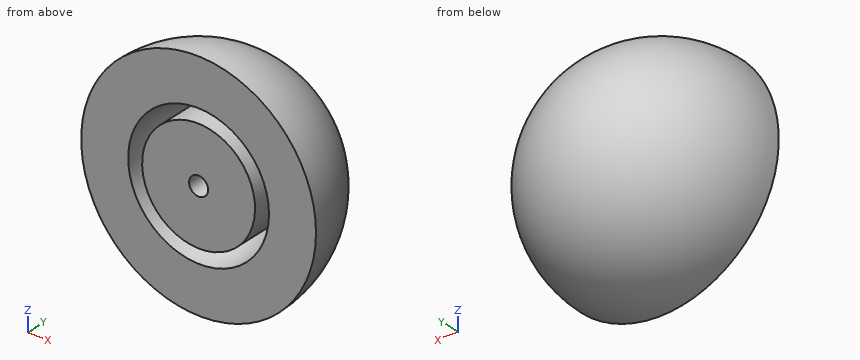
Autodesk Inventor part; units mm, degrees
ref_plane "YZ Plane" through (0, 0, 0) normal (1, 0, 0) x (0, 1, 0)
ref_plane "XZ Plane" through (0, 0, 0) normal (0, 1, 0) x (-1, 0, 0)
ref_plane "XY Plane" through (0, 0, 0) normal (0, 0, 1) x (1, 0, 0)
sketch "Sketch1" plane through (0, 0, 0) normal (0, 0, 1) x (1, 0, 0)
  line L0 (0, 0) -> (0, 20)
  line L1 (0, 0) -> (20, 0)
  arc A0 (20, 0) -> (0, 20) centre (0, 0) ccw
  line L2 (0, -4.8284) -> (0, 28.9706)
  dimension "d2" = 20
revolve "Revolution1" add sketch "Sketch1" angle 360 about axis through (0, -10, 0) along (0, 1, 0)
sketch "Sketch4" plane through (0, 0, 0) normal (0, -1, 0) x (1, 0, 0)
  point P0 (0, 0)
  point P1 (0, 0)
hole "Hole2" at (0, 0, 0) direction (0, 1, 0) diameter 3.242 depth 11.8 tip angle 118
shell "Shell2" thickness 8 removed faces 1 at (13.676, 0, 1.6606)
properties part number "Ball_Upper Half" material "Nylon 6/6"
The model under review builds one solid part; all positions refer to its coordinate system, in mm. Give positions to 0.01 mm unless a question says otherwise; leave off trailing zeros. Write each loop counter-clockwise with the first axis right and the second up, starting at its lowest first coordinate (ties: lowest second). Pieces come first, ordered by that corner, then holes.
1. Add section B-B, the plane z = -7. Write out the cut boundary in (x, y) (3 decimals).
2. Add section D-D, the plane y = 13.5. Write out the cut boundary in (x, z).
3. For P1, Ø10, axis at y = 9.5, z = -12, coming from the +X side; P2, Ø6, axis at x = -3, z = 10.5, coming from the +Y side; P3, Ø1.5, axis at y = 4.5, z = 11, coming from the -X side, all flat-tipped, find the tip position at first contact; note any pin that passes through.
4. Add section C-C, the plane x = -3. Write out the cut boundary in (y, z), plus the area to 3 significant figures.
5. Wall thickness on L1, parallel to Z at x = 0, y = 5; L2, parallel to X at y = 3.5, z = 0; L3, parallel to Z at x = -7, y = 3.25: over which ranges is each line inside the solid? List them lowest first.
6. Add section A-A, the plane y = 4. Write out the cut boundary in (x, z).
Worked answers:
1. outline: (-18.735, 0) - (-9.747, 0) arc R9.747 cw to (-6.6, 7.172) - (-6.6, 0) - (6.6, 0) - (6.6, 7.172) arc R9.747 cw to (9.747, 0) - (18.735, 0) arc R18.735 ccw to start
2. outline: circle Ø29.51 at (0, 0)
3. P1: stops at x = 17.14
3. P2: stops at y = 18.36
3. P3: stops at x = -16.61
4. outline: (0, -19.77) arc R19.77 ccw to (0, 19.77) - (0, 11.62) arc R11.62 cw to (7.17, 9.14) - (0, 9.14) - (0, -9.14) - (7.17, -9.14) arc R11.62 cw to (0, -11.62) - close
4. area: 590 mm2
5. L1: z = -19.36 to -10.91, -9.62 to -1.62, 1.62 to 9.62, 10.91 to 19.36
5. L2: x = -19.69 to -11.48, -9.62 to -1.62, 1.62 to 9.62, 11.48 to 19.69
5. L3: z = -18.45 to -9.19, -6.6 to 6.6, 9.19 to 18.45
6. outline: circle Ø39.19 at (0, 0); circle Ø19.24 at (0, 0); hole circle Ø22.63 at (0, 0); hole circle Ø3.24 at (0, 0)
